Design review of the part built by this model. Coordinates are the model's own, in mm. Coordinates: 2 decimals unless noted, no trailing zeros. Answer as a JSON object with one key per item and string values.
from build123d import *

# Parameters (mm, degrees)
SKETCH1_R      = 3.2639
FINALCUT_DEPTH = 965.2


with BuildPart() as part:
    # Sketch1 → FinalCut (new body)
    with BuildSketch(Plane.XY):
        with BuildLine():
            Line((-6.731, 0), (-6.731, 4.575738531))
            Line((-6.731, 4.575738531), (-12.442261469, 10.287))
            Line((-12.442261469, 10.287), (-15.6718, 10.287))
            Line((-15.6718, 10.287), (-15.6718, 6.858))
            Line((-15.6718, 6.858), (-14.478, 6.858))
            Line((-14.478, 6.858), (-14.478, 4.064))
            Line((-14.478, 4.064), (-19.05, 4.064))
            Line((-19.05, 4.064), (-19.05, 15.875))
            ThreePointArc((-19.05, 15.875), (-18.12006403, 18.12006403), (-15.875, 19.05))
            Line((-15.875, 19.05), (-4.064, 19.05))
            Line((-4.064, 19.05), (-4.064, 14.478))
            Line((-4.064, 14.478), (-6.858, 14.478))
            Line((-6.858, 14.478), (-6.858, 15.6718))
            Line((-6.858, 15.6718), (-10.287, 15.6718))
            Line((-10.287, 15.6718), (-10.287, 12.442261469))
            Line((-10.287, 12.442261469), (-4.575738531, 6.731))
            Line((-4.575738531, 6.731), (0, 6.731))
            Line((0, 6.731), (4.575738531, 6.731))
            Line((4.575738531, 6.731), (10.287, 12.442261469))
            Line((10.287, 12.442261469), (10.287, 15.6718))
            Line((10.287, 15.6718), (6.858, 15.6718))
            Line((6.858, 15.6718), (6.858, 14.478))
            Line((6.858, 14.478), (4.064, 14.478))
            Line((4.064, 14.478), (4.064, 19.05))
            Line((4.064, 19.05), (15.875, 19.05))
            ThreePointArc((15.875, 19.05), (18.12006403, 18.12006403), (19.05, 15.875))
            Line((19.05, 15.875), (19.05, 4.064))
            Line((19.05, 4.064), (14.478, 4.064))
            Line((14.478, 4.064), (14.478, 6.858))
            Line((14.478, 6.858), (15.6718, 6.858))
            Line((15.6718, 6.858), (15.6718, 10.287))
            Line((15.6718, 10.287), (12.442261469, 10.287))
            Line((12.442261469, 10.287), (6.731, 4.575738531))
            Line((6.731, 4.575738531), (6.731, 0))
            Line((6.731, 0), (6.731, -4.575738531))
            Line((6.731, -4.575738531), (12.442261469, -10.287))
            Line((12.442261469, -10.287), (15.6718, -10.287))
            Line((15.6718, -10.287), (15.6718, -6.858))
            Line((15.6718, -6.858), (14.478, -6.858))
            Line((14.478, -6.858), (14.478, -4.064))
            Line((14.478, -4.064), (19.05, -4.064))
            Line((19.05, -4.064), (19.05, -15.875))
            ThreePointArc((19.05, -15.875), (18.12006403, -18.12006403), (15.875, -19.05))
            Line((15.875, -19.05), (4.064, -19.05))
            Line((4.064, -19.05), (4.064, -14.478))
            Line((4.064, -14.478), (6.858, -14.478))
            Line((6.858, -14.478), (6.858, -15.6718))
            Line((6.858, -15.6718), (10.287, -15.6718))
            Line((10.287, -15.6718), (10.287, -12.442261469))
            Line((10.287, -12.442261469), (4.575738531, -6.731))
            Line((4.575738531, -6.731), (0, -6.731))
            Line((0, -6.731), (-4.575738531, -6.731))
            Line((-4.575738531, -6.731), (-10.287, -12.442261469))
            Line((-10.287, -12.442261469), (-10.287, -15.6718))
            Line((-10.287, -15.6718), (-6.858, -15.6718))
            Line((-6.858, -15.6718), (-6.858, -14.478))
            Line((-6.858, -14.478), (-4.064, -14.478))
            Line((-4.064, -14.478), (-4.064, -19.05))
            Line((-4.064, -19.05), (-15.875, -19.05))
            ThreePointArc((-15.875, -19.05), (-18.12006403, -18.12006403), (-19.05, -15.875))
            Line((-19.05, -15.875), (-19.05, -4.064))
            Line((-19.05, -4.064), (-14.478, -4.064))
            Line((-14.478, -4.064), (-14.478, -6.858))
            Line((-14.478, -6.858), (-15.6718, -6.858))
            Line((-15.6718, -6.858), (-15.6718, -10.287))
            Line((-15.6718, -10.287), (-12.442261469, -10.287))
            Line((-12.442261469, -10.287), (-6.731, -4.575738531))
            Line((-6.731, -4.575738531), (-6.731, 0))
        make_face()
        Circle(SKETCH1_R, mode=Mode.SUBTRACT)
        with BuildLine():
            Line((17.272, 11.8872), (17.272, 14.478))
            ThreePointArc((17.272, 14.478), (16.453656347, 16.453656347), (14.478, 17.272))
            Line((14.478, 17.272), (11.8872, 17.272))
            Line((11.8872, 17.272), (11.8872, 11.8872))
            Line((11.8872, 11.8872), (17.272, 11.8872))
        make_face(mode=Mode.SUBTRACT)
        with BuildLine():
            Line((11.8872, -11.8872), (17.272, -11.8872))
            Line((17.272, -11.8872), (17.272, -14.478))
            ThreePointArc((17.272, -14.478), (16.453656347, -16.453656347), (14.478, -17.272))
            Line((14.478, -17.272), (11.8872, -17.272))
            Line((11.8872, -17.272), (11.8872, -11.8872))
        make_face(mode=Mode.SUBTRACT)
        with BuildLine():
            Line((-17.272, -11.8872), (-17.272, -14.478))
            ThreePointArc((-17.272, -14.478), (-16.453656347, -16.453656347), (-14.478, -17.272))
            Line((-14.478, -17.272), (-11.8872, -17.272))
            Line((-11.8872, -17.272), (-11.8872, -11.8872))
            Line((-11.8872, -11.8872), (-17.272, -11.8872))
        make_face(mode=Mode.SUBTRACT)
        with BuildLine():
            Line((-11.8872, 11.8872), (-17.272, 11.8872))
            Line((-17.272, 11.8872), (-17.272, 14.478))
            ThreePointArc((-17.272, 14.478), (-16.453656347, 16.453656347), (-14.478, 17.272))
            Line((-14.478, 17.272), (-11.8872, 17.272))
            Line((-11.8872, 17.272), (-11.8872, 11.8872))
        make_face(mode=Mode.SUBTRACT)
    extrude(amount=-FINALCUT_DEPTH)


solid = part.part
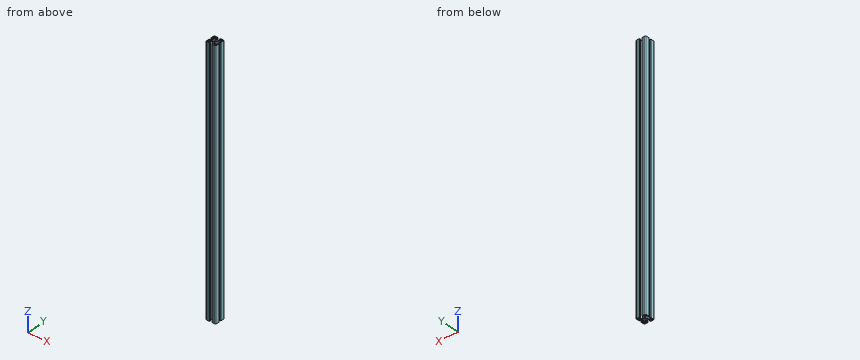
1) Insertion check: pin 1 Ø2.5 at (x, z) = (0.5, -536) entering from +Y. The pin has a flat end and moves straight along its axis. Give the tip position at first contact, or say it passes through.
Taken from the geometry:
{"pin 1": "stops at y = 6.73"}
2) Add section A-A (z = -572.5). Count the separate pieces of the cut face and the enclosed holes in it, and give its area (3 significant figures).
Taken from the geometry:
{"separate pieces": "1", "enclosed holes": "5", "area": "612 mm2"}
3) To check wall thickness, follow L1, parallel to X at y = 12.5, z = -553; L2, parallel to Y at x = -0.5, z = -713. State the ranges of each line that lie inside material, in increasing order.
Taken from the geometry:
{"L1": "x = -19.05 to -17.27, -11.89 to -10.29, 10.29 to 11.89, 17.27 to 19.05", "L2": "y = -6.73 to -3.23, 3.23 to 6.73"}
